from build123d import *

# Parameters (mm, degrees)
SKETCH_1_W          = 35
SKETCH_1_H          = 70
EXTRUDE_1_DEPTH     = 12
CUT_EXTRUDE_1_REACH = 81.177
SKETCH_3_W          = 20
SKETCH_3_H          = 70
CUT_EXTRUDE_2_DEPTH = 79.574805122


with BuildPart() as part:
    # 草图1 → 凸台-拉伸1 (new body)
    with BuildSketch(Plane.XY):
        with Locations((17.5, -35)):
            Rectangle(SKETCH_1_W, SKETCH_1_H)
    extrude(amount=EXTRUDE_1_DEPTH)

    # 草图2 → 切除-拉伸1 (cut, up to next)
    with BuildSketch(Plane.XZ.offset(70), mode=Mode.PRIVATE) as cut_extrude_1_sk1:
        Polygon((28.5, 7.328862426), (28.5, 5), (0, 5), (0, 12), (25, 12), (25, 11.5), align=None)
    cut_extrude_1_tool1 = extrude(cut_extrude_1_sk1.sketch, amount=-CUT_EXTRUDE_1_REACH, mode=Mode.PRIVATE) & part.part
    add(cut_extrude_1_tool1.solids().sort_by_distance((13.633689, -70, 8.408444))[0], mode=Mode.SUBTRACT)

    # 草图3 → 切除-拉伸2 (cut, through all)
    with BuildSketch(Plane.XY.offset(5)):
        with Locations((10, -35)):
            Rectangle(SKETCH_3_W, SKETCH_3_H)
    extrude(amount=-CUT_EXTRUDE_2_DEPTH, mode=Mode.SUBTRACT)


solid = part.part
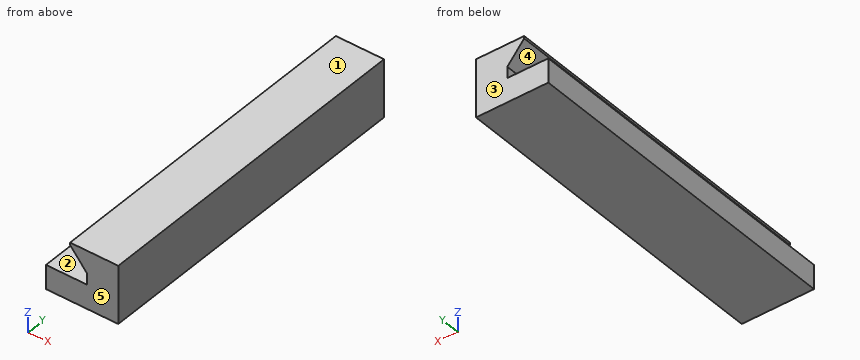
The listing builds one solid part. Answer for the finished solid, in the listing's coordinates (mm). Face numbers are marked on the shaded views. A direction names the side the tool comes from. Give positions to 0.01 mm unless a question says otherwise; leave off trailing zeros. Loops run counter-clockwise (first coordinate to the right, second up) from the corner with the lowest first, then second, coordinate; pieces in that order, holes last.
Item 1: A cutting plane is placed at A-A (x = 26.5). Give the vertices of the cut face in (y, z), then the cut area to 3 significant figures.
Derived:
outline: (-70, 0) - (0, 0) - (0, 5) - (-70, 5) - close; (-70, 9.71) - (0, 9.71) - (0, 12) - (-70, 12) - close
area: 510 mm2
Item 2: A tool of negligible diameter and unlimited length cuts with its end or side. For the marked faces 4 and 5, from which of +Z, -Z, +X, -X, +Y, -Y can it reach the whole face along a straight path? Write none if from no direction.
Derived:
face 4: -X, +Y, -Y
face 5: +Z, -Z, +X, -X, -Y
Item 3: A cutting plane is placed at D-D (z = 9.5). Give the vertices of the cut face in (x, y).
Derived:
outline: (26.68, -70) - (35, -70) - (35, 0) - (26.68, 0) - close
Item 4: A cutting plane is placed at C-C (x = 23.5). Give the vertices of the cut face in (y, z), then the cut area to 3 significant figures.
Derived:
outline: (-70, 0) - (0, 0) - (0, 5) - (-70, 5) - close
area: 350 mm2
Item 5: Each of these flat-tipped pins is pushed along its axis until it touches: pin 1 Ø1.5 at (y, z) = (-60, 10) entering from -X; pin 2 Ø7 at (x, y) = (23, -49.5) entering from +Z; pin 3 Ø3 at (y, z) = (-32.5, 7.5) entering from -X; pin 4 Ø1.2 at (y, z) = (-32, 6.5) entering from -X. Where does it stop, or does it pass through?
Derived:
pin 1: stops at x = 25.63
pin 2: stops at z = 12
pin 3: stops at x = 27.1
pin 4: stops at x = 28.5
Item 6: Determine the mould class of the marked faces 1, 2 and 3 for opening direction Z: +Z half, -Z half, draft (parallel to the pull), parting line (faces both ways), or undercut.
Derived:
face 1: +Z half
face 2: undercut
face 3: draft
Item 7: A cutting plane is placed at B-B (y = -34). Give the vertices of the cut face in (x, z), then the cut area to 3 significant figures.
Derived:
outline: (20, 0) - (35, 0) - (35, 12) - (25, 12) - (25, 11.5) - (28.5, 7.33) - (28.5, 5) - (20, 5) - close
area: 130 mm2
Item 8: Find the intervals of material crossed by line 1 along Z through (x, y) = (23, -52); line 2 along X through (y, z) = (-9, 7); line 3 along Z through (x, y) = (28, -59), in increasing order.
Derived:
line 1: z = 0 to 5
line 2: x = 28.5 to 35
line 3: z = 0 to 5, 7.92 to 12
